```python
from build123d import *

# Parameters (mm, degrees)
SKETCH_1_W               = 90
SKETCH_1_H               = 1.3
SKETCH_2_R               = 2.5
EXTRUDE_1_DEPTH          = 10
EXTRUDE_START            = 10
SKETCH_3_R               = 2.5
EXTRUDE_2_DEPTH          = 10
EXTRUDE_3_DEPTH          = 1
EXTRUDE_3_DEPTH_BACK     = 1
SKETCH_4_R               = 1.55
EXTRUDE_4_DEPTH          = 2.5
EXTRUDE_4_DEPTH_BACK     = 2.5
SKETCH_5_R               = 2.5
CHAMFER_1_SIZE           = 3
CHAMFER_1_SIZE_2         = 1.732050808
FILLET_1_R               = 2.5
CUT_EXTRUDE_1_DEPTH      = 109.936146208
CUT_EXTRUDE_1_DEPTH_BACK = 109.936146208
SKETCH_6_R               = 1.5


with BuildPart() as part:
    # 草图1 → 旋转1 (revolve)
    with BuildSketch(Plane.XY, mode=Mode.PRIVATE) as revolve_1_sk:
        with Locations((45, 0.65)):
            Rectangle(SKETCH_1_W, SKETCH_1_H)
    revolve(revolve_1_sk.sketch.rotate(Axis((0, 0, 0), (1, 0, 0)), 90), axis=Axis((0, 0, 0), (1, 0, 0)))

    # 草图2 → 凸台-拉伸1 (add)
    with BuildSketch(Plane(origin=(90, 0, 0), x_dir=(0, 0, -1), z_dir=(1, 0, 0))):
        Circle(SKETCH_2_R)
    extrude(amount=EXTRUDE_1_DEPTH)

    # 草图3 → 凸台-拉伸2 (add)
    with BuildSketch(Plane.ZY.offset(EXTRUDE_START)):
        with Locations(Location((0, 0, 0), (0, 0, 180))):
            Circle(SKETCH_3_R)
    extrude(amount=-EXTRUDE_2_DEPTH)

    # 草图4 → 凸台-拉伸3 (add, two sides: drawn at the far end of the back side and taken through both)
    # profile 1 of 2: a face of its own
    with BuildSketch(Plane.XY.offset(-EXTRUDE_3_DEPTH_BACK)):
        with BuildLine():
            Line((100, 2.5), (100, -2.5))
            Line((100, -2.5), (105, -3.839745962))
            ThreePointArc((105, -3.839745962), (108.839745962, 0), (105, 3.839745962))
            Line((105, 3.839745962), (100, 2.5))
        make_face()
        with Locations((105, 0)):
            Circle(SKETCH_4_R, mode=Mode.SUBTRACT)
    # profile 2 of 2: a face of its own
    with BuildSketch(Plane.XY.offset(-EXTRUDE_3_DEPTH_BACK)):
        with BuildLine():
            Line((-10, 2.5), (-15, 3.839745962))
            ThreePointArc((-15, 3.839745962), (-18.839745962, 0), (-15, -3.839745962))
            Line((-15, -3.839745962), (-10, -2.5))
            Line((-10, -2.5), (-10, 2.5))
        make_face()
        with Locations((-15, 0)):
            Circle(SKETCH_4_R, mode=Mode.SUBTRACT)
    extrude(amount=EXTRUDE_3_DEPTH + EXTRUDE_3_DEPTH_BACK)

    # 草图5 → 凸台-拉伸4 (add, two sides: drawn at the far end of the back side and taken through both)
    with BuildSketch(Plane.XY.offset(-EXTRUDE_4_DEPTH_BACK)):
        with Locations((105, 0)):
            Circle(SKETCH_5_R)
        with Locations((-15, 0)):
            Circle(SKETCH_5_R)
    extrude(amount=EXTRUDE_4_DEPTH + EXTRUDE_4_DEPTH_BACK)

    # 倒角1
    # the kernel refuses this chamfer: 3, 1.732050808 mm, written as the material it takes off along each edge
    with BuildSketch(Plane(origin=(100, 0, 0), x_dir=(0, 0, -1), z_dir=(0, -1, 0))) as chamfer_1_piece_1_section:
        Polygon((2.5, -CHAMFER_1_SIZE), (2.5 - CHAMFER_1_SIZE_2, 0), (2.5, 0), align=None)
    chamfer_1_piece_1 = revolve(axis=Axis((100, 0, 0), (1, 0, 0)), revolution_arc=244.335649535, mode=Mode.PRIVATE)
    chamfer_1_piece_1 = split(chamfer_1_piece_1, bisect_by=Plane(origin=(98.91025403, 0.96255065, -1), z_dir=(0, 0, -1)), keep=Keep.TOP, mode=Mode.PRIVATE)
    add(chamfer_1_piece_1, mode=Mode.SUBTRACT)
    with BuildSketch(Plane(origin=(100, 0, 0), x_dir=(0, 0, -1), z_dir=(0, -1, 0))) as chamfer_1_piece_2_section:
        Polygon((2.5, -CHAMFER_1_SIZE), (2.5 - CHAMFER_1_SIZE_2, 0), (2.5, 0), align=None)
    chamfer_1_piece_2 = revolve(axis=Axis((100, 0, 0), (1, 0, 0)), revolution_arc=244.335649535, mode=Mode.PRIVATE)
    chamfer_1_piece_2 = split(chamfer_1_piece_2, bisect_by=Plane(origin=(98.892055311, -0.028025322, 1), z_dir=(0, 0, 1)), keep=Keep.TOP, mode=Mode.PRIVATE)
    add(chamfer_1_piece_2, mode=Mode.SUBTRACT)
    with BuildSketch(Plane(origin=(100, 0, 0), x_dir=(0, 0.003141587485879368, -0.9999950652018581), z_dir=(0, -0.9999950652018581, -0.003141587485879368))) as chamfer_1_piece_3_section:
        Polygon((2.5, -CHAMFER_1_SIZE), (2.5 - CHAMFER_1_SIZE_2, 0), (2.5, 0), align=None)
    chamfer_1_piece_3 = revolve(axis=Axis((100, 0, 0), (1, 0, 0)), revolution_arc=359.64, mode=Mode.PRIVATE)
    chamfer_1_piece_3 = split(chamfer_1_piece_3, bisect_by=Plane(origin=(98.910233235, 0.965609903, -1), z_dir=(0, 0, -1)), keep=Keep.TOP, mode=Mode.PRIVATE)
    add(chamfer_1_piece_3, mode=Mode.SUBTRACT)
    with BuildSketch(Plane(origin=(100, 0, 0), x_dir=(0, 0.003141587485879368, -0.9999950652018581), z_dir=(0, -0.9999950652018581, -0.003141587485879368))) as chamfer_1_piece_4_section:
        Polygon((2.5, -CHAMFER_1_SIZE), (2.5 - CHAMFER_1_SIZE_2, 0), (2.5, 0), align=None)
    chamfer_1_piece_4 = revolve(axis=Axis((100, 0, 0), (1, 0, 0)), revolution_arc=359.64, mode=Mode.PRIVATE)
    chamfer_1_piece_4 = split(chamfer_1_piece_4, bisect_by=Plane(origin=(98.91025403, -2e-09, 1), z_dir=(0, 0, 1)), keep=Keep.TOP, mode=Mode.PRIVATE)
    add(chamfer_1_piece_4, mode=Mode.SUBTRACT)
    with BuildSketch(Plane(origin=(-10, 0, 0), x_dir=(0, 0, -1), z_dir=(0, 1, 0))) as chamfer_1_piece_5_section:
        Polygon((2.5, -CHAMFER_1_SIZE), (2.5 - CHAMFER_1_SIZE_2, 0), (2.5, 0), align=None)
    chamfer_1_piece_5 = revolve(axis=Axis((-10, 0, 0), (-1, 0, 0)), revolution_arc=244.335649535, mode=Mode.PRIVATE)
    chamfer_1_piece_5 = split(chamfer_1_piece_5, bisect_by=Plane(origin=(-8.91025403, -0.96255065, -1), z_dir=(0, 0, -1)), keep=Keep.TOP, mode=Mode.PRIVATE)
    add(chamfer_1_piece_5, mode=Mode.SUBTRACT)
    with BuildSketch(Plane(origin=(-10, 0, 0), x_dir=(0, 0, -1), z_dir=(0, 1, 0))) as chamfer_1_piece_6_section:
        Polygon((2.5, -CHAMFER_1_SIZE), (2.5 - CHAMFER_1_SIZE_2, 0), (2.5, 0), align=None)
    chamfer_1_piece_6 = revolve(axis=Axis((-10, 0, 0), (-1, 0, 0)), revolution_arc=244.335649535, mode=Mode.PRIVATE)
    chamfer_1_piece_6 = split(chamfer_1_piece_6, bisect_by=Plane(origin=(-8.892055311, 0.028025322, 1), z_dir=(0, 0, 1)), keep=Keep.TOP, mode=Mode.PRIVATE)
    add(chamfer_1_piece_6, mode=Mode.SUBTRACT)
    with BuildSketch(Plane(origin=(-10, 0, 0), x_dir=(0, -0.0031415874858794677, -0.9999950652018581), z_dir=(0, 0.9999950652018581, -0.0031415874858794677))) as chamfer_1_piece_7_section:
        Polygon((2.5, -CHAMFER_1_SIZE), (2.5 - CHAMFER_1_SIZE_2, 0), (2.5, 0), align=None)
    chamfer_1_piece_7 = revolve(axis=Axis((-10, 0, 0), (-1, 0, 0)), revolution_arc=359.64, mode=Mode.PRIVATE)
    chamfer_1_piece_7 = split(chamfer_1_piece_7, bisect_by=Plane(origin=(-8.910233235, -0.965609903, -1), z_dir=(0, 0, -1)), keep=Keep.TOP, mode=Mode.PRIVATE)
    add(chamfer_1_piece_7, mode=Mode.SUBTRACT)
    with BuildSketch(Plane(origin=(-10, 0, 0), x_dir=(0, -0.0031415874858794677, -0.9999950652018581), z_dir=(0, 0.9999950652018581, -0.0031415874858794677))) as chamfer_1_piece_8_section:
        Polygon((2.5, -CHAMFER_1_SIZE), (2.5 - CHAMFER_1_SIZE_2, 0), (2.5, 0), align=None)
    chamfer_1_piece_8 = revolve(axis=Axis((-10, 0, 0), (-1, 0, 0)), revolution_arc=359.64, mode=Mode.PRIVATE)
    chamfer_1_piece_8 = split(chamfer_1_piece_8, bisect_by=Plane(origin=(-8.91025403, 2e-09, 1), z_dir=(0, 0, 1)), keep=Keep.TOP, mode=Mode.PRIVATE)
    add(chamfer_1_piece_8, mode=Mode.SUBTRACT)
    with BuildSketch(Plane(origin=(-10, 0, 0), x_dir=(0, -0.901346670332976, 0.43309834896898114), z_dir=(0, -0.43309834896898114, -0.901346670332976))) as chamfer_1_piece_9_section:
        Polygon((2.5, -CHAMFER_1_SIZE), (2.5 - CHAMFER_1_SIZE_2, 0), (2.5, 0), align=None)
    chamfer_1_piece_9 = revolve(axis=Axis((-10, 0, 0), (-1, 0, 0)), revolution_arc=244.335649535, mode=Mode.PRIVATE)
    chamfer_1_piece_9 = split(chamfer_1_piece_9, bisect_by=Plane(origin=(-8.89205531, -0.028025322, 1), z_dir=(0, 0, 1)), keep=Keep.TOP, mode=Mode.PRIVATE)
    add(chamfer_1_piece_9, mode=Mode.SUBTRACT)
    with BuildSketch(Plane(origin=(-10, 0, 0), x_dir=(0, -0.901346670332976, 0.43309834896898114), z_dir=(0, -0.43309834896898114, -0.901346670332976))) as chamfer_1_piece_10_section:
        Polygon((2.5, -CHAMFER_1_SIZE), (2.5 - CHAMFER_1_SIZE_2, 0), (2.5, 0), align=None)
    chamfer_1_piece_10 = revolve(axis=Axis((-10, 0, 0), (-1, 0, 0)), revolution_arc=244.335649535, mode=Mode.PRIVATE)
    chamfer_1_piece_10 = split(chamfer_1_piece_10, bisect_by=Plane(origin=(-8.910254031, 0.96255065, -1), z_dir=(0, 0, -1)), keep=Keep.TOP, mode=Mode.PRIVATE)
    add(chamfer_1_piece_10, mode=Mode.SUBTRACT)
    with BuildSketch(Plane(origin=(100, 0, 0), x_dir=(0, 0.9013466703329771, 0.43309834896897925), z_dir=(0, 0.43309834896897925, -0.9013466703329771))) as chamfer_1_piece_11_section:
        Polygon((2.5, -CHAMFER_1_SIZE), (2.5 - CHAMFER_1_SIZE_2, 0), (2.5, 0), align=None)
    chamfer_1_piece_11 = revolve(axis=Axis((100, 0, 0), (1, 0, 0)), revolution_arc=244.335649535, mode=Mode.PRIVATE)
    chamfer_1_piece_11 = split(chamfer_1_piece_11, bisect_by=Plane(origin=(98.89205531, 0.028025322, 1), z_dir=(0, 0, 1)), keep=Keep.TOP, mode=Mode.PRIVATE)
    add(chamfer_1_piece_11, mode=Mode.SUBTRACT)
    with BuildSketch(Plane(origin=(100, 0, 0), x_dir=(0, 0.9013466703329771, 0.43309834896897925), z_dir=(0, 0.43309834896897925, -0.9013466703329771))) as chamfer_1_piece_12_section:
        Polygon((2.5, -CHAMFER_1_SIZE), (2.5 - CHAMFER_1_SIZE_2, 0), (2.5, 0), align=None)
    chamfer_1_piece_12 = revolve(axis=Axis((100, 0, 0), (1, 0, 0)), revolution_arc=244.335649535, mode=Mode.PRIVATE)
    chamfer_1_piece_12 = split(chamfer_1_piece_12, bisect_by=Plane(origin=(98.910254031, -0.96255065, -1), z_dir=(0, 0, -1)), keep=Keep.TOP, mode=Mode.PRIVATE)
    add(chamfer_1_piece_12, mode=Mode.SUBTRACT)

    # 圆角1
    # the kernel refuses this fillet: 2.5 mm, written as the material it takes off along each edge
    with BuildSketch(Plane(origin=(105, 0, -2.5), x_dir=(1, 0, 0), z_dir=(0, -1, 0))) as fillet_1_piece_1:
        with BuildLine():
            CenterArc((0.208712153, 2.5), FILLET_1_R, 270, 66.421821522)
            Line((0.208712153, 0), (0.208712153, -0.05))
            Line((0.208712153, -0.05), (2.5, -0.05))
            Line((2.5, -0.05), (2.55, 0))
            ThreePointArc((2.55, 0), (2.55, 0.75), (2.545825757, 1.48))
            Line((2.545825757, 1.48), (2.5, 1.5))
        make_face()
    revolve(axis=Axis((105, 0, -2.5), (0, 0, 1)), mode=Mode.SUBTRACT)
    with BuildSketch(Plane(origin=(105, 0, 2.5), x_dir=(1, 0, 0), z_dir=(0, -1, 0))) as fillet_1_piece_2:
        with BuildLine():
            CenterArc((0.208712153, -2.5), FILLET_1_R, 23.578178478, 66.421821522)
            Line((0.208712153, 0), (0.208712153, 0.05))
            Line((0.208712153, 0.05), (2.5, 0.05))
            Line((2.5, 0.05), (2.55, 0))
            ThreePointArc((2.55, 0), (2.55, -0.75), (2.545825757, -1.48))
            Line((2.545825757, -1.48), (2.5, -1.5))
        make_face()
    revolve(axis=Axis((105, 0, 2.5), (0, 0, 1)), mode=Mode.SUBTRACT)
    with BuildSketch(Plane(origin=(-15, 0, -2.5), x_dir=(1, 0, 0), z_dir=(0, -1, 0))) as fillet_1_piece_3:
        with BuildLine():
            CenterArc((0.208712153, 2.5), FILLET_1_R, 270, 66.421821522)
            Line((0.208712153, 0), (0.208712153, -0.05))
            Line((0.208712153, -0.05), (2.5, -0.05))
            Line((2.5, -0.05), (2.55, 0))
            ThreePointArc((2.55, 0), (2.55, 0.75), (2.545825757, 1.48))
            Line((2.545825757, 1.48), (2.5, 1.5))
        make_face()
    revolve(axis=Axis((-15, 0, -2.5), (0, 0, 1)), mode=Mode.SUBTRACT)
    with BuildSketch(Plane(origin=(-15, 0, 2.5), x_dir=(1, 0, 0), z_dir=(0, -1, 0))) as fillet_1_piece_4:
        with BuildLine():
            CenterArc((0.208712153, -2.5), FILLET_1_R, 23.578178478, 66.421821522)
            Line((0.208712153, 0), (0.208712153, 0.05))
            Line((0.208712153, 0.05), (2.5, 0.05))
            Line((2.5, 0.05), (2.55, 0))
            ThreePointArc((2.55, 0), (2.55, -0.75), (2.545825757, -1.48))
            Line((2.545825757, -1.48), (2.5, -1.5))
        make_face()
    revolve(axis=Axis((-15, 0, 2.5), (0, 0, 1)), mode=Mode.SUBTRACT)

    # 草图6 → 切除-拉伸1 (cut, two sides: drawn at the far end of the back side and taken through both)
    with BuildSketch(Plane.XY.offset(-CUT_EXTRUDE_1_DEPTH_BACK)):
        with Locations((-15, 0)):
            Circle(SKETCH_6_R)
        with Locations(Location((105, 0, 0), (0, 0, 180))):
            Circle(SKETCH_6_R)
    extrude(amount=CUT_EXTRUDE_1_DEPTH + CUT_EXTRUDE_1_DEPTH_BACK, mode=Mode.SUBTRACT)


solid = part.part
```
Model file for the job. Use its own axes, mm. A direction names the side the tool comes from. Round coordinates to 2 decimals unless told otherwise and drop trailing zeros. Write each loop counter-clockwise with the first axis right and the second up, starting at its lowest first coordinate (ties: lowest second). Pieces come first, ordered by that corner, then holes. Notation, with made-up numbers: (83, 65) -> (104, 65) arc R17 ccw to (104, 72) -> close; hole circle Ø2 at (23, 71.5). An arc over 180 degrees is marked (long way). Answer as CSV lines item,"result".
1. Pin check, flat tips, straight feed: pin 1 Ø3 at (y, z) = (-2, 0) entering from +X; pin 2 Ø4 at (x, y) = (-15, 0) entering from -Z; pin 3 Ø4 at (x, y) = (-15.5, 1.5) entering from +Z. Stop position of each tip, or through.
Resolved:
pin 1,"x = 108.81"
pin 2,"z = -2.14"
pin 3,"z = 2.14"
2. Slice it at A-A, the plane x = 25. List the corners of the cut face in (y, z).
Resolved:
outline,"circle Ø2.6 at (0, 0)"
3. Tool access for faces 1 (the face through (-13, -2, 1)), 2 (the face through (-12.46, 3.16, -0.01)), 3 (the face through (-8.317, 0.028, -1.739)), 4 (the face through (102.46, -3.16, -0.01)), 5 (the face through (45.63, -1.29, -0.17)): list every direction of +Z, -Z, +X, -X, +Y, -Y with a clear straight run to the whole face (end or side of a thin tool).
Resolved:
face 1,"+Z"
face 2,"+Z, -Z, +Y"
face 3,"-Z"
face 4,"+Z, -Z, -Y"
face 5,"none"
4. Mould opens along X. For faces 6 (the face through (102.54, 3.18, -0.01)), 7 (the face through (108.84, -0.08, -0.01)), 8 (the face through (-13, -2, -1)), 9 (the face through (-18.84, 0.08, -0.01)) say: +X half, -X half, draft (parallel to the pull), parting line (faces both ways), or undercut.
Resolved:
face 6,"undercut"
face 7,"+X half"
face 8,"undercut"
face 9,"-X half"
5. Drill centre lines: line 1 (X direction, y = 0.25, z = 0.8); line 2 (X direction, y = -0.75, z = 1.65); line 3 (X direction, y = 0.5, z = 1.4). Where is each one in solid material? Low to high.
Resolved:
line 1,"-18.83 to -16.48, -13.52 to 103.52, 106.48 to 108.83"
line 2,"-16.95 to -16.3, -13.7 to -13.05, -8.19 to 0, 90 to 98.19, 103.05 to 103.7, 106.3 to 106.95"
line 3,"-17.22 to -16.41, -13.59 to -12.78, -8.76 to 0, 90 to 98.76, 102.78 to 103.59, 106.41 to 107.22"
